```python
from build123d import *

# Parameters (mm, degrees)
SKETCH1_W                      = 82
SKETCH1_H                      = 208
BOSS_EXTRUDE1_DEPTH            = 1
F_3_2_3_2_DIAMETER_HOLE1_D     = 3.2
F_3_2_3_2_DIAMETER_HOLE1_DEPTH = 1
SKETCH7_W                      = 50
SKETCH7_H                      = 20
CUT_EXTRUDE2_DEPTH             = 10
F_2_5_2_5_DIAMETER_HOLE1_D     = 2.5
F_1_75_1_75_DIAMETER_HOLE1_D   = 1.75
SKETCH12_R                     = 1.25
CUT_EXTRUDE3_DEPTH             = 10
SKETCH13_R                     = 5.614838764
CUT_EXTRUDE4_DEPTH             = 10


with BuildPart() as part:
    # Sketch1 → Boss-Extrude1 (new body)
    with BuildSketch(Plane.XY):
        Rectangle(SKETCH1_W, SKETCH1_H)
    extrude(amount=BOSS_EXTRUDE1_DEPTH)

    # Ø3.2 (3.2) Diameter Hole1
    with Locations(Plane.XY.offset(1)):
        with Locations((-30.5, 10), (30.5, 10), (30.49999746, -100.29999968), (-30.50000246, -100.29999968), (-30.5, 101.3), (30.5, 101.3), (30.49999746, -8.7), (30.644996947, -118.559802529), (-30.50000246, -8.7)):
            Hole(F_3_2_3_2_DIAMETER_HOLE1_D / 2, depth=F_3_2_3_2_DIAMETER_HOLE1_DEPTH)

    # Sketch7 → Cut-Extrude2 (cut)
    with BuildSketch(Plane(origin=(0, 0, 0), x_dir=(-1, 0, 0), z_dir=(0, 0, -1))):
        with Locations((-1, -22)):
            Rectangle(SKETCH7_W, SKETCH7_H)
        with Locations((1, 24)):
            Rectangle(SKETCH7_W, SKETCH7_H)
    extrude(amount=-CUT_EXTRUDE2_DEPTH, mode=Mode.SUBTRACT)

    # Ø2.5 (2.5) Diameter Hole1 (through all)
    with Locations(Plane(origin=(0, 0, 0), x_dir=(-1, 0, 0), z_dir=(0, 0, -1))):
        with Locations((-29, -80.702796173), (-38.5, -80.702796173)):
            Hole(F_2_5_2_5_DIAMETER_HOLE1_D / 2)

    # Ø1.75 (1.75) Diameter Hole1 (through all)
    with Locations(Plane.XY.offset(1)):
        with Locations((-25.1, 0.65), (-11.6, 0.65)):
            Hole(F_1_75_1_75_DIAMETER_HOLE1_D / 2)

    # Sketch12 → Cut-Extrude3 (cut)
    with BuildSketch(Plane.XY.offset(1)):
        with Locations((-8, -2.84999878)):
            Circle(SKETCH12_R)
        with Locations((11.75, -2.84999878)):
            Circle(SKETCH12_R)
        with Locations((11.75, 4.15000122)):
            Circle(SKETCH12_R)
    extrude(amount=-CUT_EXTRUDE3_DEPTH, mode=Mode.SUBTRACT)

    # Sketch13 → Cut-Extrude4 (cut)
    with BuildSketch(Plane(origin=(0, 0, 0), x_dir=(-1, 0, 0), z_dir=(0, 0, -1))):
        with Locations((-2.25, 0.65000122)):
            Circle(SKETCH13_R)
    extrude(amount=-CUT_EXTRUDE4_DEPTH, mode=Mode.SUBTRACT)


solid = part.part
```
Here's how the part is built. I have some questions about the finished solid (model axes, mm). Give positions to 0.01 mm unless a question says otherwise; leave off trailing zeros. Order: outer loops, then holes, each group sorted by start corner. A loop starts at its lowest first (then second) coordinate and runs counter-clockwise, first axis right, second up. Notation, with made-up numbers: (17.5, 74.25) -> (71.5, 74.25) arc R30 cw to (71.5, 107.25) -> close; hole circle Ø8 at (25.5, -22). An arc over 180 degrees is marked (long way). Use CSV: the item, a comma, the result in double quotes. Start each with the question number.
Item 1: Suppose I cut it at A-A (x = 2.25). List the corners of the cut face in (y, z) for me.
Item 2: I'm going to push a flat-ended pin straight in: P1, Ø1.5, axis at x = -8, y = -2.85, coming from the -Z side. Where does the tip first touch, or does it pass through?
Item 3: If I drill on probe 1 along Y at (x, z) = (-5.5, 0.2); probe 2 along Y at (x, z) = (2.25, 0.45); probe 3 along Y at (x, z) = (11.75, 0.6), over which ranges is the centre line in solid material (lowest first)? Write a range as [from, to].
Item 4: Thinking about a two-plate mould opening in X: for faces 1 (the cylindrical face through (3.47, -4.83, 0.49)), 2 (the flat face through (-10, 1, 1)), which applies, pulls with the +X half, pulls with the -X half, needs draft (parallel to the pull), parting line crosses it, or undercut?
Item 5: Suppose I cut it at B-B (z = 0.65). Give the number of separate pieces and of enclosed holes in the cut face, and give its area (3 significant figures).
Answer block:
1,outline,"(-104, 0) -> (-32, 0) -> (-32, 1) -> (-104, 1) -> close; (-12, 0) -> (-4.96, 0) -> (-4.96, 1) -> (-12, 1) -> close; (6.26, 0) -> (14, 0) -> (14, 1) -> (6.26, 1) -> close; (34, 0) -> (104, 0) -> (104, 1) -> (34, 1) -> close"
2,P1,"passes through"
3,probe 1,"y = [-104, -32], [-12, 14], [34, 104]"
3,probe 2,"y = [-104, -32], [-12, -4.96], [6.26, 14], [34, 104]"
3,probe 3,"y = [-104, -32], [-12, -4.1], [-1.6, 2.9], [5.4, 14], [34, 104]"
4,face 1,"undercut"
4,face 2,"needs draft"
5,separate pieces,"1"
5,enclosed holes,"18"
5,area,"14,900 mm^2"
